Can you work these out from the model? Positions are in its coordinate system, mm. Give positions to 0.01 mm unless a question says otherwise; leave off trailing zeros. Loops run counter-clockwise (first coordinate to the right, second up) from the corner with the lowest first, then second, coordinate; pieces in that order, holes last.
from build123d import *

# Parameters (mm, degrees)
F0_W     = 87.64372
F0_H     = 88.9
F1_DEPTH = 25.4
F3_DEPTH = 25.4
F4_DEPTH = 25.4


with BuildPart() as f1:
    # F0 (on Top) → F1 (new body)
    with BuildSketch(Plane.XY):
        Rectangle(F0_W, F0_H)
    extrude(amount=F1_DEPTH)

    # F2 (on face) → F3 (join)
    with BuildSketch(Plane.XY.offset(25.4)):
        with BuildLine():
            ThreePointArc((-23.397237, 22.612818), (-27.638216, 22.533643), (-23.39658, 22.560036))
            ThreePointArc((-23.39658, 22.560036), (-23.396744, 22.586429), (-23.397237, 22.612818))
        make_face()
    extrude(amount=F3_DEPTH)

    # F2 (on face) → F4 (join)
    with BuildSketch(Plane.XY.offset(25.4)):
        with BuildLine():
            ThreePointArc((-22.260667, -23.069627), (-22.260831, -23.043234), (-22.261324, -23.016845))
            ThreePointArc((-22.261324, -23.016845), (-26.502303, -23.09602), (-22.260667, -23.069627))
        make_face()
    extrude(amount=F4_DEPTH)


solid = f1.part
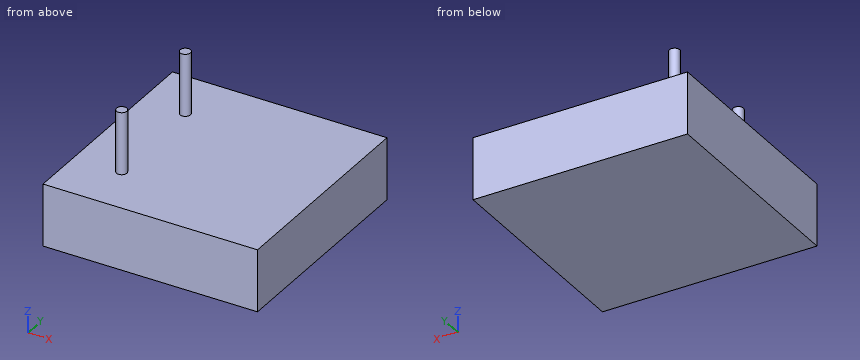
(1) Suppose I cut it at C-C on y = 29. List the corners of the cut face in (x, z) for me.
Returned:
outline: (-43.82, 0) - (43.82, 0) - (43.82, 25.4) - (-43.82, 25.4) - close
(2) Will this pin go through, and if not, where does the flat tip stop? P1, Ø6, axis at x = 20, y = -13, coming from the +Z side.
Returned:
P1: stops at z = 25.4
(3) Please list where these lines run through material, in increasing order: probe 1 along Z at (x, y) = (-17, -6.5); probe 2 along Y at (x, z) = (-27, 42).
Returned:
probe 1: z = 0 to 25.4
probe 2: y = 21.04 to 24.08
(4) Suppose I cut it at A-A on z = 43. List the corners of the cut face in (x, y) for me, plus the area to 3 significant figures.
Returned:
outline: (-23.4, 22.56) arc R2.12 ccw to (-23.4, 22.61) arc R2.12 ccw (long way) to start; (-22.26, -23.07) arc R2.12 ccw to (-22.26, -23.02) arc R2.12 ccw (long way) to start
area: 28.3 mm2
(5) Suppose I cut it at B-B on x = -31. List the corners of the cut face in (y, z) for me, plus the area to 3 significant figures.
Returned:
outline: (-44.45, 0) - (44.45, 0) - (44.45, 25.4) - (-44.45, 25.4) - close
area: 2,260 mm2
